Check sheet for the modelled part. Datum: model origin and axes. Units: mm. A direction names the side the tool comes from. Give positions to 0.01 mm unless a question says otherwise; leave off trailing zeros. Loops run counter-clockwise (first coordinate to the right, second up) from the corner with the lowest first, then second, coordinate; pieces in that order, holes last. Notation, with made-up numbers: (6.25, -16) -> (56.25, -16) arc R34 cw to (56.25, 20) -> close; hole circle Ø2 at (-1.5, 70). An arc over 180 degrees is marked (long way). Answer as CSV lines item,"result". Start each with the question number.
(1) Gauge pin test, flat ends, axial feed: pin 1 Ø3 at (x, z) = (57.5, 59) entering from -Y; pin 2 Ø10 at (x, y) = (88, -1.5) entering from -Z; pin 3 Ø7 at (x, y) = (86, 0.5) entering from +Z; pin 4 Ø3 at (x, z) = (-10, 40) entering from -Y. Record the tip position at first contact, or that the pin passes through.
(2) Release check for a two-part mould opening along X. For faces 1 (the face through (100, 2, 39)), 2 (the face through (40, -18, 35)), 3 (the face through (90, 3, 80)) record: pulls with the +X half, pulls with the -X half, needs draft (parallel to the pull), parting line crosses it, or undercut.
(3) Material ranges on line 1 (Z direction, x = -10, y = 1.45); line 2 (Z direction, x = 54, y = 6.5), recorded low to high. Write a range as from..to.
(4) Access from +Z, -Z, +X, -X, +Y, -Y to the whole of each face (thin tool, end or side, straight path). Record for faces 4 (the face through (39, 15, 0)), 5 (the face through (94, 0, 39)), 6 (the face through (40.49, 0.437, 42.535)), 7 (the face through (39.83, -13.99, 120.87)), 8 (the face through (41, -45, 39)).
(5) Section check B-B on z = 70. Enter the section's corners in (x, y), plus the area to 3 significant figures.
(6) Section check A-A on x = -10. Enter the section's corners in (y, z).
(7) Section check C-C on z = 22.5. Enter the section's corners in (x, y).
from build123d import *

# Parameters (mm, degrees)
EXTRUDE_1_DEPTH     = 80
SKETCH_4_R          = 2.6
CUT_EXTRUDE_2_DEPTH = 150
CHAMFER_1_SIZE      = 4
CHAMFER_2_SIZE      = 4
SKETCH_8_W          = 70
SKETCH_8_H          = 70
CUT_EXTRUDE_3_DEPTH = 70
EXTRUDE_3_DEPTH     = 80
EXTRUDE_4_DEPTH     = 80
SKETCH_25_W         = 25
SKETCH_25_H         = 25.122105301
CUT_EXTRUDE_8_DEPTH = 20


with BuildPart() as part:
    # 草图2 → 凸台-拉伸1 (new body)
    with BuildSketch(Plane.XY):
        Polygon((0, 0), (0, -45), (80, -45), (80, 0), (100, 0), (100, 5), (80, 5), (80, 25), (0, 25), (0, 5), (-20, 5), (-20, 0), align=None)
    extrude(amount=EXTRUDE_1_DEPTH)

    # 草图4 → 切除-拉伸2 (cut)
    with BuildSketch(Plane(origin=(0, 5, 0), x_dir=(1, 0, 0), z_dir=(0, 1, 0))):
        with Locations(Location((-10, -40, 0), (0, 0, 180))):
            Circle(SKETCH_4_R)
        with Locations(Location((-10, -70, 0), (0, 0, 180))):
            Circle(SKETCH_4_R)
        with Locations(Location((-10, -10, 0), (0, 0, 180))):
            Circle(SKETCH_4_R)
        with Locations(Location((90, -10, 0), (0, 0, 180))):
            Circle(SKETCH_4_R)
        with Locations(Location((90, -40, 0), (0, 0, 180))):
            Circle(SKETCH_4_R)
        with Locations(Location((90, -70, 0), (0, 0, 180))):
            Circle(SKETCH_4_R)
    extrude(amount=-CUT_EXTRUDE_2_DEPTH, mode=Mode.SUBTRACT)

    # 倒角1
    chamfer_1_edges = [part.edges().sort_by_distance(p)[0] for p in [
        (80, 0, 40),
    ]]
    chamfer(chamfer_1_edges, length=CHAMFER_1_SIZE)

    # 倒角2
    chamfer_2_edges = [part.edges().sort_by_distance(p)[0] for p in [
        (0, 0, 40),
    ]]
    chamfer(chamfer_2_edges, length=CHAMFER_2_SIZE)

    # 草图8 → 切除-拉伸3 (cut)
    with BuildSketch(Plane(origin=(0, 25, 0), x_dir=(1, 0, 0), z_dir=(0, 1, 0))):
        with Locations((40, -40)):
            Rectangle(SKETCH_8_W, SKETCH_8_H)
    extrude(amount=-CUT_EXTRUDE_3_DEPTH, mode=Mode.SUBTRACT)

    # 草图19 → 放样3 section 0
    with BuildSketch(Plane(origin=(0, 0, -50), x_dir=(-1, 0, 0), z_dir=(0, 0, -1))):
        with BuildLine():
            Line((-60, -15), (-20, -15))
            Line((-20, -15), (-20, -55))
            Line((-20, -55), (-60, -55))
            Line((-60, -55), (-60, -15))
        make_face()
    # 草图17 → 放样3 section 1
    with BuildSketch(Plane(origin=(0, 0, 0), x_dir=(-1, 0, 0), z_dir=(0, 0, -1))):
        with BuildLine():
            Line((-80, 5), (0, 5))
            Line((0, 5), (0, -45))
            Line((0, -45), (-80, -45))
            Line((-80, -45), (-80, 5))
        make_face()
    loft_3 = loft()

    # 草图22 → 凸台-拉伸3 (add)
    with BuildSketch(Plane(origin=(80, 0, 0), x_dir=(0, 0, -1), z_dir=(1, 0, 0))):
        Polygon((-80, -45), (0, -45), (0, -40), (-40, -32), (-80, -40), align=None)
    extrude(amount=-EXTRUDE_3_DEPTH)

    # 草图20 → 切除-放样6 section 0
    with BuildSketch(Plane.XY.offset(5)):
        with BuildLine():
            Line((5, 0), (75, 0))
            Line((75, 0), (75, -40))
            Line((75, -40), (5, -40))
            Line((5, -40), (5, 0))
        make_face()
    # 草图21 → 切除-放样6 section 1
    with BuildSketch(Plane(origin=(0, 0, -50), x_dir=(-1, 0, 0), z_dir=(0, 0, -1))):
        with BuildLine():
            Line((-57.5, -20), (-22.5, -20))
            Line((-22.5, -20), (-22.5, -50))
            Line((-22.5, -50), (-57.5, -50))
            Line((-57.5, -50), (-57.5, -20))
        make_face()
    loft_6 = loft(mode=Mode.SUBTRACT)

    # 镜向1: 放样3, 切除-放样6 across plane
    add(loft_3.mirror(Plane.XY.offset(40)))
    add(loft_6.mirror(Plane.XY.offset(40)), mode=Mode.SUBTRACT)

    # 草图23 → 凸台-拉伸4 (add)
    with BuildSketch(Plane(origin=(80, 0, 0), x_dir=(0, 0, -1), z_dir=(1, 0, 0))):
        Polygon((-45, -45), (-45, -4), (-40, 5), (-35, -4), (-35, -45), align=None)
    extrude(amount=-EXTRUDE_4_DEPTH)

    # 草图25 → 切除-拉伸8 (cut)
    with BuildSketch(Plane(origin=(0, 31.896551724, 12.75862069), x_dir=(1, 0, 0), z_dir=(0, 0.9284766908852594, 0.3713906763541038))):
        with Locations((40, -129.98223454)):
            Rectangle(SKETCH_25_W, SKETCH_25_H)
    cut_extrude_8 = extrude(amount=-CUT_EXTRUDE_8_DEPTH, mode=Mode.SUBTRACT)

    # 镜向2: 切除-拉伸8 across plane
    add(cut_extrude_8.mirror(Plane.XY.offset(40)), mode=Mode.SUBTRACT)


solid = part.part
Working result:
1,pin 1,"stops at y = -45"
1,pin 2,"stops at z = 0"
1,pin 3,"stops at z = 80"
1,pin 4,"passes through"
2,face 1,"pulls with the +X half"
2,face 2,"undercut"
2,face 3,"needs draft"
3,line 1,"z = 0..7.4, 12.6..37.4, 42.6..67.4, 72.6..80"
3,line 2,"z = 0..5, 75..80"
4,face 4,"-Z, +X, -X, +Y"
4,face 5,"+Z, -Z, +X, -Y"
4,face 6,"+Y"
4,face 7,"+Z"
4,face 8,"+X, -X, -Y"
5,outline,"(-20, 0) -> (-12.6, 0) -> (-12.6, 5) -> (-20, 5) -> close; (-7.4, 0) -> (-4, 0) -> (0, -4) -> (0, -45) -> (80, -45) -> (80, -4) -> (84, 0) -> (87.4, 0) -> (87.4, 5) -> (80, 5) -> (80, 25) -> (75, 25) -> (75, -38) -> (5, -38) -> (5, 25) -> (0, 25) -> (0, 5) -> (-7.4, 5) -> close; (92.6, 0) -> (100, 0) -> (100, 5) -> (92.6, 5) -> close"
5,area,"1,350 mm^2"
6,outline,"(0, 0) -> (5, 0) -> (5, 7.4) -> (0, 7.4) -> close; (0, 12.6) -> (5, 12.6) -> (5, 37.4) -> (0, 37.4) -> close; (0, 42.6) -> (5, 42.6) -> (5, 67.4) -> (0, 67.4) -> close; (0, 72.6) -> (5, 72.6) -> (5, 80) -> (0, 80) -> close"
7,outline,"(-20, 0) -> (-4, 0) -> (0, -4) -> (0, -45) -> (80, -45) -> (80, -4) -> (84, 0) -> (100, 0) -> (100, 5) -> (80, 5) -> (80, 25) -> (75, 25) -> (75, -35.5) -> (5, -35.5) -> (5, 25) -> (0, 25) -> (0, 5) -> (-20, 5) -> close"
